```python
from build123d import *

# Parameters (mm, degrees)
SKETCH2_R               = 20
BOSS_EXTRUDE1_DEPTH     = 6
SKETCH3_R               = 19
CUT_EXTRUDE1_DEPTH      = 11
FILLET1_R               = 0.5
SKETCH5_W               = 0.5
SKETCH5_H               = 1
SKETCH6_R               = 0.375
CUT_EXTRUDE2_DEPTH      = 21.0000001
CUT_EXTRUDE2_DEPTH_BACK = 21.0000001


with BuildPart() as part:
    # Sketch2 → Boss-Extrude1 (new body, symmetric)
    with BuildSketch(Plane(origin=(0, 0, 0), x_dir=(1, 0, 0), z_dir=(0, 1, 0))):
        Circle(SKETCH2_R)
    extrude(amount=BOSS_EXTRUDE1_DEPTH, both=True)

    # Sketch3 → Cut-Extrude1 (cut)
    with BuildSketch(Plane.XZ.offset(6)):
        Circle(SKETCH3_R)
    extrude(amount=-CUT_EXTRUDE1_DEPTH, mode=Mode.SUBTRACT)

    # Fillet1
    fillet1_edges = [part.edges().sort_by_distance(p)[0] for p in [
        (-20, 6, 0),
    ]]
    fillet(fillet1_edges, radius=FILLET1_R)

    # Sketch5 → Cut-Revolve1 (revolve, cut)
    with BuildSketch(Plane.XY):
        with Locations((19.75, 0)):
            Rectangle(SKETCH5_W, SKETCH5_H)
    revolve(axis=Axis((0, 0, 0), (0, 1, 0)), mode=Mode.SUBTRACT)

    # Sketch6 → Cut-Extrude2 (cut, two sides)
    with BuildSketch(Plane.XY) as cut_extrude2_sk:
        Circle(SKETCH6_R)
    extrude(amount=CUT_EXTRUDE2_DEPTH, mode=Mode.SUBTRACT)
    extrude(cut_extrude2_sk.sketch, amount=-CUT_EXTRUDE2_DEPTH_BACK, mode=Mode.SUBTRACT)

    # Sketch7 → Revolve1 (revolve)
    with BuildSketch(Plane.XY):
        Polygon((5.9, 5), (5.9, 1), (6.9, 1), (7.9, 5), align=None)
    revolve(axis=Axis((0, 5, 0), (0, -1, 0)))


solid = part.part
```
Geometry check sheet. Reference: the model listing, model coordinates, mm. A direction names the side the tool comes from. Coordinates: 2 decimals unless noted, no trailing zeros. Loops run counter-clockwise (first coordinate to the right, second up) from the corner with the lowest first, then second, coordinate; pieces in that order, holes last. Notation, with made-up numbers: (-26.5, 48) - (12.5, 48) arc R10 ccw to (12.5, 62) - close; hole circle Ø3 at (-19.5, -26.75). An arc over 180 degrees is marked (long way). One line per item, written item: value. Start each with the question number.
(1) Cross-section at C-C on y = -2.5. Enter the section's corners in (x, z).
(2) Depth check by flat-ended pin: P1, Ø11, axis at x = -0.5, z = -2.5, coming from the -Y side; P2, Ø3, axis at y = -3.5, z = -10, coming from the +X side; P3, Ø1.5, axis at y = 3, z = -6.5, coming from the +X side. Enter the tip coordinate at first touch or a pass-through.
(3) Cross-section at A-A on y = 2. Enter the section's corners in (x, z), plus the area to 3 significant figures.
(4) Mould release check, pull along Y, two halves, no side actions. Record for faces 4 (the cylindrical face through (-4.336, 3.035, 19.524)), 5 (the flat face through (-19.2, -0.5, 4.4)), 6 (the flat face through (18, -6, 7)): released by +Y, released by -Y, zero draft, split by the parting line, or undercut.
(5) Tool access check on faces 1 (the flat face through (0, 5, 0)), 2 (the cylindrical face through (-2.539, 0.007, -19.334)), 3 (the cylindrical face through (-4.336, -3.212, 19.524)). Record the directions out of +Z, -Z, +X, -X, +Y, -Y that give a thin tool (end or side, any length) a straight path to the whole face; none if there is none.
(6) Cross-section at B-B on z = 0. Enter the section's corners in (x, y), plus the area to 3 significant figures.
(7) Material ranges on line 1 (Y direction, x = 0, z = -19.2) (3 decimals); line 2 (Z direction, x = -0.5, y = 0); line 3 (Z direction, x = 2, y = 4.5), recorded low to high. Write a range as [from, to].
Results below:
1. outline: circle Ø40 at (0, 0); hole circle Ø38 at (0, 0)
2. P1: stops at y = 1
2. P2: stops at x = 18.1
2. P3: stops at x = 19.16
3. outline: circle Ø40 at (0, 0); circle Ø14.3 at (0, 0); hole circle Ø38 at (0, 0); hole circle Ø11.8 at (0, 0)
3. area: 174 mm2
4. face 4: zero draft
4. face 5: undercut
4. face 6: released by -Y
5. face 1: -Y
5. face 2: none
5. face 3: +Y, -Y
6. outline: (-20, -6) - (-19, -6) - (-19, 5) - (-7.9, 5) - (-6.9, 1) - (-5.9, 1) - (-5.9, 5) - (5.9, 5) - (5.9, 1) - (6.9, 1) - (7.9, 5) - (19, 5) - (19, -6) - (20, -6) - (20, -0.5) - (19.5, -0.5) - (19.5, 0.5) - (20, 0.5) - (20, 5.5) arc R0.5 ccw to (19.5, 6) - (-19.5, 6) arc R0.5 ccw to (-20, 5.5) - (-20, 0.5) - (-19.5, 0.5) - (-19.5, -0.5) - (-20, -0.5) - close
6. area: 72.9 mm2
7. line 1: y = [-6, -0.375], [0.375, 6]
7. line 2: z = [-19.49, -18.99], [18.99, 19.49]
7. line 3: z = [-19.9, -18.89], [-7.51, -5.55], [5.55, 7.51], [18.89, 19.9]
